from build123d import *

# Parameters (mm, degrees)
SKETCH_1_R          = 6
EXTRUDE_1_DEPTH     = 13
SKETCH_2_R          = 5
EXTRUDE_2_DEPTH     = 2.5
SKETCH_3_R          = 8
EXTRUDE_3_DEPTH     = 31
SKETCH_4_R          = 7.5
EXTRUDE_4_DEPTH     = 2
SKETCH_5_R          = 10
EXTRUDE_5_DEPTH     = 32
SKETCH_6_R          = 13
EXTRUDE_6_DEPTH     = 33
SKETCH_7_R          = 10
EXTRUDE_7_DEPTH     = 32
SKETCH_8_R          = 7.5
EXTRUDE_8_DEPTH     = 2
SKETCH_9_R          = 8
EXTRUDE_9_DEPTH     = 33
CUT_EXTRUDE_1_DEPTH = 3
CUT_EXTRUDE_2_DEPTH = 3
CHAMFER_1_SIZE      = 1


with BuildPart() as part:
    # 草图1 → 凸台-拉伸1 (new body)
    with BuildSketch(Plane.XY):
        Circle(SKETCH_1_R)
    extrude(amount=-EXTRUDE_1_DEPTH)

    # 草图2 → 凸台-拉伸2 (add)
    with BuildSketch(Plane(origin=(0, 0, -13), x_dir=(-1, 0, 0), z_dir=(0, 0, -1))):
        Circle(SKETCH_2_R)
    extrude(amount=EXTRUDE_2_DEPTH)

    # 草图3 → 凸台-拉伸3 (add)
    with BuildSketch(Plane(origin=(0, 0, -15.5), x_dir=(-1, 0, 0), z_dir=(0, 0, -1))):
        Circle(SKETCH_3_R)
    extrude(amount=EXTRUDE_3_DEPTH)

    # 草图4 → 凸台-拉伸4 (add)
    with BuildSketch(Plane(origin=(0, 0, -46.5), x_dir=(-1, 0, 0), z_dir=(0, 0, -1))):
        Circle(SKETCH_4_R)
    extrude(amount=EXTRUDE_4_DEPTH)

    # 草图5 → 凸台-拉伸5 (add)
    with BuildSketch(Plane(origin=(0, 0, -48.5), x_dir=(-1, 0, 0), z_dir=(0, 0, -1))):
        Circle(SKETCH_5_R)
    extrude(amount=EXTRUDE_5_DEPTH)

    # 草图6 → 凸台-拉伸6 (add)
    with BuildSketch(Plane(origin=(0, 0, -80.5), x_dir=(-1, 0, 0), z_dir=(0, 0, -1))):
        Circle(SKETCH_6_R)
    extrude(amount=EXTRUDE_6_DEPTH)

    # 草图7 → 凸台-拉伸7 (add)
    with BuildSketch(Plane(origin=(0, 0, -113.5), x_dir=(-1, 0, 0), z_dir=(0, 0, -1))):
        Circle(SKETCH_7_R)
    extrude(amount=EXTRUDE_7_DEPTH)

    # 草图8 → 凸台-拉伸8 (add)
    with BuildSketch(Plane(origin=(0, 0, -145.5), x_dir=(-1, 0, 0), z_dir=(0, 0, -1))):
        Circle(SKETCH_8_R)
    extrude(amount=EXTRUDE_8_DEPTH)

    # 草图9 → 凸台-拉伸9 (add)
    with BuildSketch(Plane(origin=(0, 0, -147.5), x_dir=(-1, 0, 0), z_dir=(0, 0, -1))):
        Circle(SKETCH_9_R)
    extrude(amount=EXTRUDE_9_DEPTH)

    # 草图11 → 切除-拉伸1 (cut)
    with BuildSketch(Plane(origin=(8, 0, 0), x_dir=(0, 0, -1), z_dir=(1, 0, 0))):
        with BuildLine():
            Line((24, 2.5), (39, 2.5))
            ThreePointArc((39, 2.5), (41.5, 0), (39, -2.5))
            Line((39, -2.5), (24, -2.5))
            ThreePointArc((24, -2.5), (21.5, 0), (24, 2.5))
        make_face()
    extrude(amount=-CUT_EXTRUDE_1_DEPTH, mode=Mode.SUBTRACT)

    # 草图12 → 切除-拉伸2 (cut)
    with BuildSketch(Plane(origin=(0, -8, 0), x_dir=(1, 0, 0), z_dir=(0, 1, 0))):
        with BuildLine():
            Line((-2.5, 168), (-2.5, 153))
            ThreePointArc((-2.5, 153), (0, 150.5), (2.5, 153))
            Line((2.5, 153), (2.5, 168))
            ThreePointArc((2.5, 168), (0, 170.5), (-2.5, 168))
        make_face()
    extrude(amount=CUT_EXTRUDE_2_DEPTH, mode=Mode.SUBTRACT)

    # 草图18 → 切除-旋转1 (revolve, cut)
    with BuildSketch(Plane(origin=(0, 0, 0), x_dir=(0, 0, -1), z_dir=(1, 0, 0))):
        Polygon((149.5, 8), (152.5, 8), (152.5, 6.267949192), align=None)
    revolve(axis=Axis((0, 8, -152.5), (0, -1, 0)), mode=Mode.SUBTRACT)

    # 倒角1
    chamfer_1_edges = [part.edges().sort_by_distance(p)[0] for p in [
        (-6, 0, 0),
        (8, 0, -180.5),
    ]]
    chamfer(chamfer_1_edges, length=CHAMFER_1_SIZE)


solid = part.part
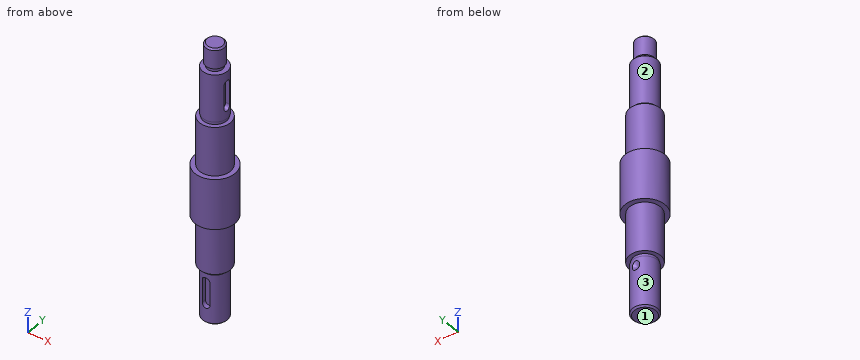
Read the model definition and answer for the solid it produces. Units are mm, in the model's axes. Face numbers are marked on the shaded views. A direction names the side the tool comes from. Coordinates: 2 decimals unless noted, no trailing zeros. Write each loop counter-clockwise with the first axis right and the second up, starting at its lowest first coordinate (ties: lowest second). Pieces come first, ordered by that corner, then holes. Notation, with made-up numbers: (54, 74.5) - (98, 74.5) arc R20 cw to (98, 113.5) - close; hole circle Ø4 at (-22.75, 86). An arc over 180 degrees is marked (long way). One line per question, with ' | ' between items.
Q1. Each of these flat-tipped pins is pushed along its axis until it touches: P1, Ø1.5, axis at y = -1, z = -27.5, coming from the +X side; P2, Ø10, axis at x = -2, z = -158, coming from the -Y side; P3, Ø6, axis at y = -4, z = -74, coming from the +X side. Where does it stop, or does it pass through?
Result set:
P1: x = 5 | P2: y = -7.6 | P3: x = 9.95
Q2. Find section A-A, the plane z = -28. Write down the section's boundary in (x, y).
Result set:
outline: (5, -2.5) - (5, 2.5) - (7.6, 2.5) arc R8 ccw (long way) to (7.6, -2.5) - close
Q3. Consider L1, parallel to Z at x = 3.25, y = -5; L2, parallel to Z at x = -6.75, y = 4; L3, parallel to Z at x = -10.5, y = -4.25. Determine where each line is inside the solid, lowest interval first. Write a range as [from, to].
Result set:
L1: [-180.5, -15.5], [-13, -0.96] | L2: [-179.65, -147.5], [-145.5, -48.5], [-46.5, -15.5] | L3: [-113.5, -80.5]
Q4. For the marked faces 1, 2 and 3, determine the directions among +Z, -Z, +X, -X, +Y, -Y from which every point of the face is accessible in a straight line to the end or side of a thin tool.
Result set:
face 1: -Z, +X, -X, +Y, -Y | face 2: +Z | face 3: -Z
Q5. Find section B-B, the plane z = -129.5. Write down the section's boundary in (x, y).
Result set:
outline: circle Ø20 at (0, 0)
